For this review, take the finished solid that the model builds, in its own axes (mm). A direction names the side the tool comes from. Give positions to 0.01 mm unless a question says otherwise; leave off trailing zeros. Order: outer loops, then holes, each group sorted by start corner. A loop starts at its lowest first (then second) coordinate and runs counter-clockwise, first axis right, second up.
Item 1: The part is to be moulded in two halves that separate along X. For faces 5 (the flat face through (-2, 2, 0)), 6 (the flat face through (2.75, 5, 3)), 7 (the flat face through (8.3, 0, 5)), say which applies: released by +X, released by -X, zero draft, split by the parting line, or undercut.
Item 2: Consider section C-C (z = 6.25). Give the boundary of the cut face in (x, y).
Item 3: Machinability: for faces 1 (the cylindrical face through (-0.195, -3.61, 1.763)), 2 (the flat face through (0, 3.507, 8)), 3 (the flat face through (0, 8.3, 5)), 4 (the flat face through (0, -5, 6.5)), which of the approach directions +Z, -Z, +X, -X, +Y, -Y give a long, thin tool a straight path to every point of the face, cutting with its end or side? Answer none if there is none.
Item 4: For probe 1 along Y at (x, z) = (0, 5.3); probe 2 along X at (y, z) = (-3.6, 3.25); probe 3 along Y at (x, z) = (-0.75, 1.5), list the stretches that pass through material, from the lowest coordinate up.
Item 5: Consider section A-A (z = 3.25). Give the boundary of the cut face in (x, y).
Item 6: Consider section D-D (x = 0). Give the number of separate pieces and of enclosed holes in the cut face, plus the area to 3 significant figures.
Item 7: Consider section B-B (y = 0.25). Give the boundary of the cut face in (x, z), plus the area to 3 significant figures.
Item 8: For P1, Ø3, axis at x = 0, y = 0, coming from the +Z side; P2, Ø1.5, axis at x = 0, y = 5, coming from the -Z side; P3, Ø0.7, axis at x = 0, y = -6, coming from the -Z side, all flat-tipped, find the tip position at first contact; note any pin that passes through.
```python
from build123d import *

# Parameters (mm, degrees)
CYLINDER_R        = 2
CYLINDER_DEPTH    = 10
PAD001_DEPTH      = 3.5
BOX_W             = 2.4
BOX_H             = 5.5
BOX_DEPTH         = 6.5
CYLINDER003_R     = 1.5
CYLINDER003_DEPTH = 5.4
CYLINDER001_R     = 1.5
CYLINDER001_DEPTH = 6
SKETCH002_W       = 5.5
SKETCH002_H       = 6
PAD002_DEPTH      = 1.2
SKETCH_W          = 16.6
SKETCH_H          = 16.6
PAD_DEPTH         = 10


with BuildPart() as cylinder:
    # Cylinder → Cylinder (new body)
    with BuildSketch(Plane.XY):
        Circle(CYLINDER_R)
    extrude(amount=CYLINDER_DEPTH)


with BuildPart() as fusion001:
    # Sketch001 → Pad001 (new body)
    with BuildSketch(Plane.XY):
        Polygon((-4.05, 0), (-2.025, -3.507403), (2.025, -3.507403), (4.05, 0), (2.025, 3.507403), (-2.025, 3.507403), align=None)
    extrude(amount=PAD001_DEPTH)


with BuildPart() as fusion001_1:
    # Body001 placement: moved
    add(fusion001.part.moved(Location((0, 0, 6.5))))

    # Fusion001: union Cylinder
    add(cylinder.part)


with BuildPart() as cube:
    # Box → Box (new body)
    with BuildSketch(Plane(origin=(-2.75, -4.5, 0), x_dir=(0, -1, 0), z_dir=(0, 0, 1))):
        with Locations((1.2, 2.75)):
            Rectangle(BOX_W, BOX_H)
    extrude(amount=BOX_DEPTH)


with BuildPart() as fusion:
    # Cylinder003 → Cylinder003 (new body)
    with BuildSketch(Plane(origin=(0, -8.5, 3.25), x_dir=(1, 0, 0), z_dir=(0, 1, 0))):
        Circle(CYLINDER003_R)
    extrude(amount=CYLINDER003_DEPTH)

    # Fusion: union Cube
    add(cube.part)


with BuildPart() as fusion_1:
    # Fusion placement: moved
    add(fusion.part.moved(Location((0, 0.2, 0))))


with BuildPart() as cylinder001:
    # Cylinder001 → Cylinder001 (new body)
    with BuildSketch(Plane(origin=(0, 3, -3), x_dir=(1, 0, 0), z_dir=(0, 0, 1))):
        Circle(CYLINDER001_R)
    extrude(amount=CYLINDER001_DEPTH)


with BuildPart() as fusion003:
    # Sketch002 → Pad002 (new body, symmetric)
    with BuildSketch(Plane.XY):
        with Locations((0, 3)):
            Rectangle(SKETCH002_W, SKETCH002_H)
    extrude(amount=PAD002_DEPTH, both=True)

    # Fusion002: union Cylinder001
    add(cylinder001.part)


with BuildPart() as fusion003_1:
    # Fusion002 placement: moved
    add(fusion003.part.moved(Location((0, 2.3, 3))))

    # Fusion003: union Fusion001, Fusion
    add(fusion001_1.part)
    add(fusion_1.part)


with BuildPart() as cut:
    # Sketch → Pad (new body)
    with BuildSketch(Plane.XY):
        Rectangle(SKETCH_W, SKETCH_H)
    extrude(amount=PAD_DEPTH)

    # Cut: cut Fusion003
    add(fusion003_1.part, mode=Mode.SUBTRACT)


solid = cut.part
```
Resolved:
1. face 5: zero draft
1. face 6: undercut
1. face 7: released by +X
2. outline: (-8.3, -8.3) - (8.3, -8.3) - (8.3, 8.3) - (-8.3, 8.3) - close; hole (-2.75, -6.7) - (2.75, -6.7) - (2.75, -4.3) - (-2.75, -4.3) - close; hole circle Ø4 at (0, 0)
3. face 1: -Y
3. face 2: +Z
3. face 3: +Z, -Z, +X, -X, +Y
3. face 4: -Z
4. probe 1: y = -8.3 to -6.7, -4.3 to -2, 2 to 3.8, 6.8 to 8.3
4. probe 2: x = -8.3 to -1.5, 1.5 to 8.3
4. probe 3: y = -8.3 to -6.7, -4.3 to -1.85, 1.85 to 4, 6.6 to 8.3
5. outline: (-8.3, -8.3) - (-1.5, -8.3) - (-1.5, -6.7) - (-2.75, -6.7) - (-2.75, -4.3) - (-1.5, -4.3) - (-1.5, -2.9) - (1.5, -2.9) - (1.5, -4.3) - (2.75, -4.3) - (2.75, -6.7) - (1.5, -6.7) - (1.5, -8.3) - (8.3, -8.3) - (8.3, 8.3) - (2.75, 8.3) - (2.75, 2.3) - (-2.75, 2.3) - (-2.75, 8.3) - (-8.3, 8.3) - close; hole circle Ø4 at (0, 0)
6. separate pieces: 4
6. enclosed holes: 0
6. area: 65.6 mm2
7. outline: (-8.3, 0) - (-1.98, 0) - (-1.98, 6.5) - (-3.91, 6.5) - (-3.91, 10) - (-8.3, 10) - close; (1.98, 0) - (8.3, 0) - (8.3, 10) - (3.91, 10) - (3.91, 6.5) - (1.98, 6.5) - close
7. area: 113 mm2
8. P1: passes through
8. P2: stops at z = 6
8. P3: stops at z = 6.5
